Input: dimensioned drawing with shaded views. Units: mm. Origin: part minimum x, y, z. Round coordinates to 2 decimals unless told otherwise and drop trailing zeros. Loops run counter-clockwise (first coordinate to the right, second up) from the corner with the lowest first, then second, coordinate; pieces in that order, holes last. Notation, with made-up numbers: (-24, 62) -> (32, 62) arc R11 ccw to (32, 79) -> close; hole circle Ø4 at (82, 64). An arc over 180 degrees is marked (long way). Answer as a JSON object with one key per item and string values.
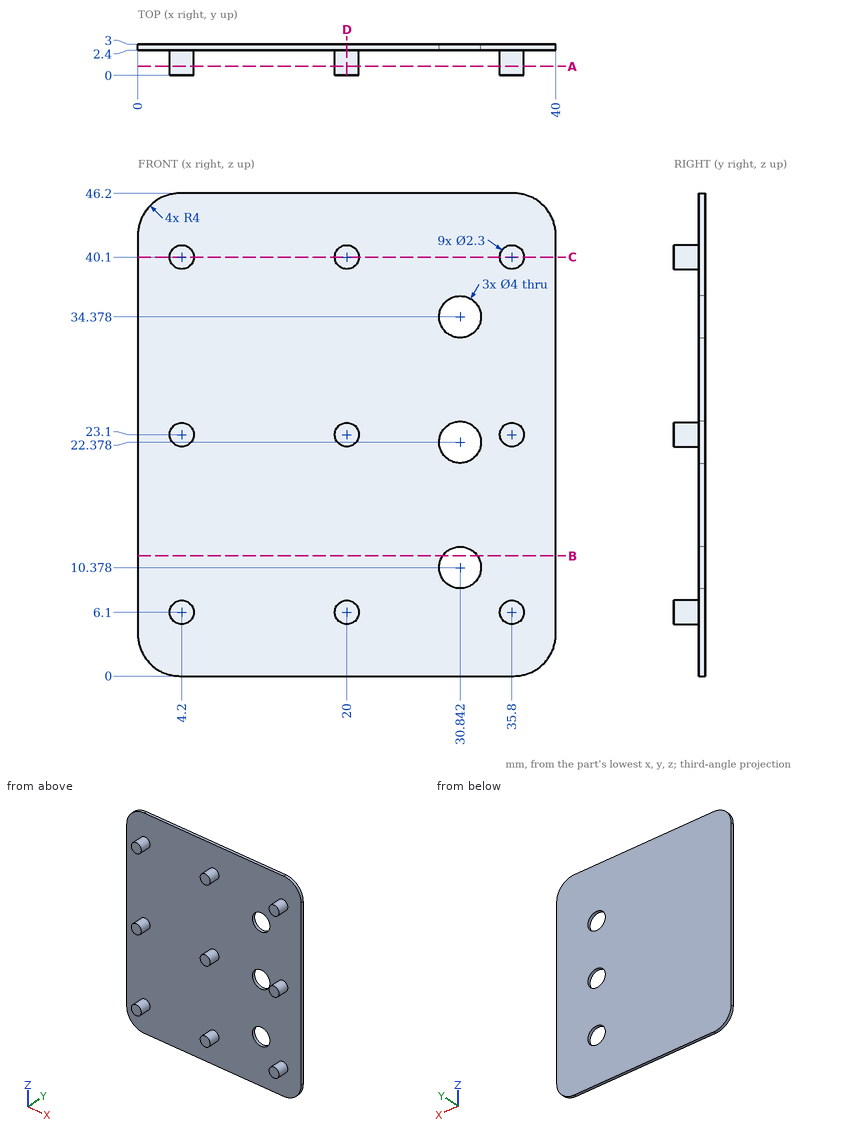
1) Section D-D, the plane x = 20. Output: boundary loops of the cut face in (y, z).
Output:
{"outline": "(0, 4.95) -> (2.4, 4.95) -> (2.4, 0) -> (3, 0) -> (3, 46.2) -> (2.4, 46.2) -> (2.4, 41.25) -> (0, 41.25) -> (0, 38.95) -> (2.4, 38.95) -> (2.4, 24.25) -> (0, 24.25) -> (0, 21.95) -> (2.4, 21.95) -> (2.4, 7.25) -> (0, 7.25) -> close"}
2) Contact query for a flat-ended pin moving along its axis: P1, Ø1.5, axis at y = 0.5, z = 21.5, coming from the +X side (1 decimal). Output: stop coordinate, or through.
Output:
{"P1": "stops at x = 36.6"}
3) Section C-C, the plane z = 40.1. Output: boundary loops of the cut face in (x, y).
Output:
{"outline": "(0, 2.4) -> (3.05, 2.4) -> (3.05, 0) -> (5.35, 0) -> (5.35, 2.4) -> (18.85, 2.4) -> (18.85, 0) -> (21.15, 0) -> (21.15, 2.4) -> (34.65, 2.4) -> (34.65, 0) -> (36.95, 0) -> (36.95, 2.4) -> (40, 2.4) -> (40, 3) -> (0, 3) -> close"}
4) Ray query, probe 1 along X at (y, z) = (1.4, 24) (1 decimal); probe 2 along Z at (x, y) = (19.5, 1.25) (1 decimal); probe 3 along Z at (x, y) = (30, 2.55) (1 decimal). Return the intervals inside material, ascending.
Output:
{"probe 1": "x = 3.5 to 4.9, 19.3 to 20.7, 35.1 to 36.5", "probe 2": "z = 5.1 to 7.1, 22.1 to 24.1, 39.1 to 41.1", "probe 3": "z = 0 to 8.6, 12.2 to 20.6, 24.2 to 32.6, 36.2 to 46.2"}
5) Section A-A, the plane y = 0.85. Count the separate pieces of the cut face and the enclosed holes in it.
Output:
{"separate pieces": "9", "enclosed holes": "0"}
6) Section B-B, the plane z = 11.5. Output: boundary loops of the cut face in (x, y).
Output:
{"outline": "(0, 2.4) -> (29.19, 2.4) -> (29.19, 3) -> (0, 3) -> close; (32.5, 2.4) -> (40, 2.4) -> (40, 3) -> (32.5, 3) -> close"}
